For this review, take the finished solid that the model builds, in its own axes (mm). Face numbers are marked on the shaded views. A direction names the side the tool comes from. Round coordinates to 2 decimals unless told otherwise and drop trailing zeros. Write each loop counter-clockwise with the first axis right and the second up, starting at its lowest first coordinate (ties: lowest second). Pieces come first, ordered by that corner, then holes.
from build123d import *

# Parameters (mm, degrees)
CROQUIS1_R              = 3.175
CROQUIS1_R_2            = 1.5875
SALIENTE_EXTRUIR1_DEPTH = 3.81
CROQUIS2_W              = 12.70653568
CROQUIS2_H              = 6.35
CORTAR_EXTRUIR1_DEPTH   = 20.32
CROQUIS3_W              = 6.35
CROQUIS3_H              = 7.62
CORTAR_EXTRUIR2_DEPTH   = 20.32
CROQUIS4_W              = 3.81
CROQUIS4_H              = 1.27
CORTAR_EXTRUIR3_DEPTH   = 20.32
CROQUIS5_R              = 1.5875
CORTAR_EXTRUIR4_DEPTH   = 53.34
CORTAR_EXTRUIR6_DEPTH   = 53.34


with BuildPart() as part:
    # Croquis1 → Saliente-Extruir1 (new, symmetric)
    with BuildSketch(Plane.XY):
        with BuildLine():
            Line((-5.602941176, -2.988235294), (-3.175, -12.7))
            ThreePointArc((-3.175, -12.7), (0, -15.875), (3.175, -12.7))
            Line((3.175, -12.7), (5.602941176, -2.988235294))
            ThreePointArc((5.602941176, -2.988235294), (0, 6.35), (-5.602941176, -2.988235294))
        make_face()
        with Locations(Location((0, 0, 0), (0, 0, 180))):
            Circle(CROQUIS1_R, mode=Mode.SUBTRACT)
        with Locations(Location((0, -12.7, 0), (0, 0, 180))):
            Circle(CROQUIS1_R_2, mode=Mode.SUBTRACT)
    extrude(amount=SALIENTE_EXTRUIR1_DEPTH, both=True)

    # Croquis2 → Cortar-Extruir1 (cut)
    with BuildSketch(Plane(origin=(0, 0, 0), x_dir=(1, 0, 0), z_dir=(0, 1, 0))):
        with Locations((0.00326784, 0)):
            Rectangle(CROQUIS2_W, CROQUIS2_H)
    extrude(amount=-CORTAR_EXTRUIR1_DEPTH, mode=Mode.SUBTRACT)

    # Croquis3 → Cortar-Extruir2 (cut)
    with BuildSketch(Plane(origin=(0, 0, 0), x_dir=(0, 0, -1), z_dir=(1, 0, 0))):
        with Locations((0, 3.81)):
            Rectangle(CROQUIS3_W, CROQUIS3_H)
    extrude(amount=CORTAR_EXTRUIR2_DEPTH, mode=Mode.SUBTRACT)

    # Croquis4 → Cortar-Extruir3 (cut)
    with BuildSketch(Plane(origin=(0, 0, 0), x_dir=(0, 0, -1), z_dir=(1, 0, 0))):
        with Locations((-1.905, 2.315882353)):
            Rectangle(CROQUIS4_W, CROQUIS4_H)
    extrude(amount=-CORTAR_EXTRUIR3_DEPTH, mode=Mode.SUBTRACT)

    # Croquis5 → Cortar-Extruir4 (cut)
    with BuildSketch(Plane(origin=(0, 0, 0), x_dir=(1, 0, 0), z_dir=(0, 1, 0))):
        Circle(CROQUIS5_R)
    extrude(amount=CORTAR_EXTRUIR4_DEPTH, mode=Mode.SUBTRACT)

    # Croquis6 → Cortar-Extruir6 (cut)
    with BuildSketch(Plane(origin=(0, 0, 0), x_dir=(1, 0, 0), z_dir=(0, 1, 0))):
        Polygon((0, 0), (-5.622703384, 0), (-6.123490387, 0), (-6.123490387, 0.508), (0, 0.508), align=None)
    extrude(amount=CORTAR_EXTRUIR6_DEPTH, mode=Mode.SUBTRACT)


solid = part.part
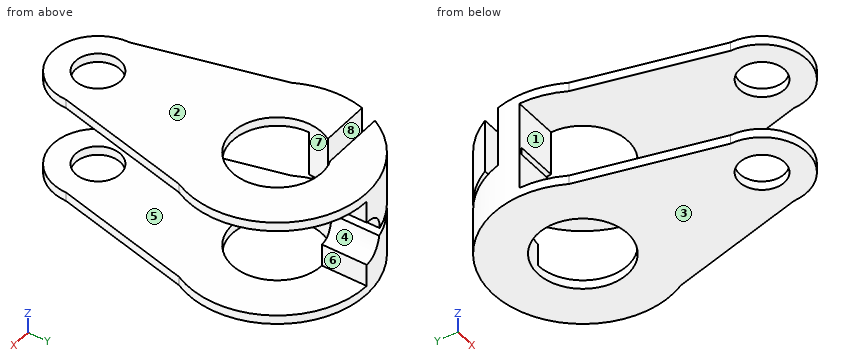
(1) For the marked faces 1, 2, 3, 4 and 5, list the 3-axis set-ups (+Z, -Z, +X, -X, +Y, -Y) from which the entire face can be reached by the end or side of a thin tool; tool diameter is ignored.
Geometry check:
face 1: +X, -X, -Y
face 2: +Z, +X, -X, +Y, -Y
face 3: -Z, +X, -X, +Y, -Y
face 4: +X, +Y, -Y
face 5: +X, -Y
(2) For line 1 along Z through (x, y) = (5.75, 2) (3 decimals); line 2 along X through (y, z) = (-12.7, -3.4) (1 decimal); line 3 along X through (y, z) = (-2.25, -3.5), list the stretches that pass through material, from the lowest coordinate up.
Geometry check:
line 1: z = -3.81 to -3.175, 3.175 to 3.81
line 2: x = -3.2 to -1.6, 1.6 to 3.2
line 3: x = -5.94 to -2.24, 2.24 to 5.94
(3) We need section B-B, the plane x = -4.25. Give the boundary of the cut face in (y, z) (3 decimals).
Geometry check:
outline: (-8.4, -3.81) - (4.718, -3.81) - (4.718, -0.508) - (0, -0.508) - (0, -3.175) - (-8.4, -3.175) - close; (-8.4, 3.175) - (0, 3.175) - (0, 0) - (1.681, 0) - (1.681, 3.81) - (-8.4, 3.81) - close; (2.951, 0) - (4.718, 0) - (4.718, 3.81) - (2.951, 3.81) - close
(4) Mouldability with a two-part tool opening along X and no side actions: class the marked faces 6, 7 and 8 as pulls with the +X half, pulls with the -X half, needs draft (parallel to the pull), parting line crosses it, or undercut.
Geometry check:
face 6: pulls with the +X half
face 7: undercut
face 8: needs draft
(5) For pin 1 Ø4 at (y, z) = (3.5, 2) entering from -X; pin 2 Ø1.3 at (y, z) = (4.5, 2) entering from +X; pin 3 Ø4 at (x, z) = (-5, 2.5) entering from +Y, all flat-tipped, find the tip position at first contact; note any pin that passes through.
Geometry check:
pin 1: stops at x = -6.17
pin 2: stops at x = 0
pin 3: stops at y = 5.6
(6) We need section A-A, the plane y = -10.25. Give the boundary of the cut face in (x, z) (1 decimal), and give its area (3 significant figures).
Geometry check:
outline: (-3.8, -3.8) - (3.8, -3.8) - (3.8, -3.2) - (-3.8, -3.2) - close; (-3.8, 3.2) - (3.8, 3.2) - (3.8, 3.8) - (-3.8, 3.8) - close
area: 9.62 mm2
(7) We need section D-D, the plane x = 4.25. Give the boundary of the cut face in (y, z) (3 decimals), and give its area (3 significant figures).
Geometry check:
outline: (-8.4, -3.81) - (4.718, -3.81) - (4.718, -3.175) - (-8.4, -3.175) - close; (-8.4, 3.175) - (4.718, 3.175) - (4.718, 3.81) - (-8.4, 3.81) - close
area: 16.7 mm2
(8) We need section C-C, the plane z = -3.5. State how many separate pieces and enclosed holes the cut face has, and give its area (3 significant figures).
Geometry check:
separate pieces: 1
enclosed holes: 2
area: 161 mm2
